Job drawing, mm, ordinate dimensions from the low corner. One solid piece. Give positions to 0.01 mm unless a question says otherwise; leave off trailing zeros. Order: outer loops, then holes, each group sorted by start corner. A loop starts at its lowest first (then second) coordinate and runs counter-clockwise, first axis right, second up.
Item 1: Band-saw the part on D-D on z = 0.5. Give the cut face in (x, y), plus the area to 3 significant figures.
Item 2: Band-saw the part on A-A on z = 3.5. Give the cut face in (x, y), plus the area to 3 significant figures.
Item 3: Wall check: L1, parallel to Z at x = 3.5, y = 1.7; L2, parallel to X at y = 2.5, z = 2.75; L3, parallel to X at y = 0.1, z = 2.5. Give the ranges that are in metal, low to high.
Item 4: Band-saw the part on B-B on x = 56.5. Give the cut face in (y, z), plus the area to 3 significant figures.
Item 5: Band-saw the part on C-C on y = 2. Give the cut face in (x, z), plus the area to 3 significant figures.
Item 6: Flat gauge pins, fed straight in: P1, Ø1.5, axis at y = 1.5, z = 2, coming from the -X side; P2, Ø1, axis at x = 26.5, y = 1.5, coming from the -Z side; P3, Ø1.4, axis at x = 35, y = 1.5, coming from the +Z side. Where does each tip first touch, or does it go through?
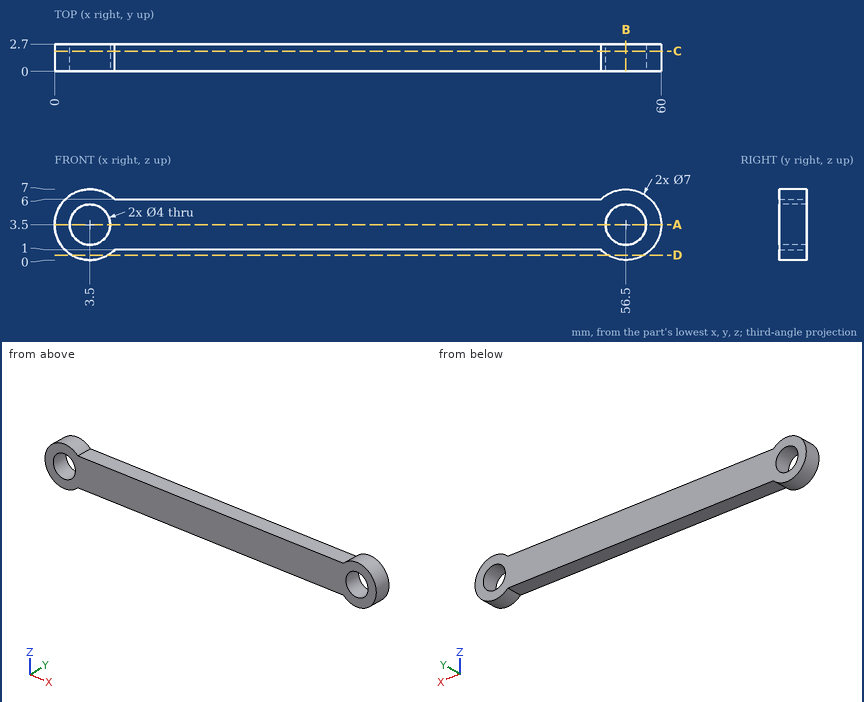
The answers:
1. outline: (1.7, 0) - (5.3, 0) - (5.3, 2.7) - (1.7, 2.7) - close; (54.7, 0) - (58.3, 0) - (58.3, 2.7) - (54.7, 2.7) - close
1. area: 19.5 mm2
2. outline: (0, 0) - (1.5, 0) - (1.5, 2.7) - (0, 2.7) - close; (5.5, 0) - (54.5, 0) - (54.5, 2.7) - (5.5, 2.7) - close; (58.5, 0) - (60, 0) - (60, 2.7) - (58.5, 2.7) - close
2. area: 140 mm2
3. L1: z = 0 to 1.5, 5.5 to 7
3. L2: x = 0.08 to 1.65, 5.35 to 54.65, 58.35 to 59.92
3. L3: x = 0.15 to 1.77, 5.23 to 54.77, 58.23 to 59.85
4. outline: (0, 0) - (2.7, 0) - (2.7, 1.5) - (0, 1.5) - close; (0, 5.5) - (2.7, 5.5) - (2.7, 7) - (0, 7) - close
4. area: 8.10 mm2
5. outline: (5.95, 1) - (54.05, 1) arc R3.5 ccw (long way) to (54.05, 6) - (5.95, 6) arc R3.5 ccw (long way) to start; hole circle Ø4 at (3.5, 3.5); hole circle Ø4 at (56.5, 3.5)
5. area: 285 mm2
6. P1: stops at x = 0.08
6. P2: stops at z = 1
6. P3: stops at z = 6
